```python
from build123d import *

# Parameters (mm, degrees)
SKETCH1_W           = 212.725
SKETCH1_H           = 185.42
BOSS_EXTRUDE1_DEPTH = 3.175
SKETCH5_W           = 3.175
SKETCH5_H           = 76.2
BOSS_EXTRUDE2_DEPTH = 3.175
SKETCH6_W           = 76.2
SKETCH6_H           = 3.175
BOSS_EXTRUDE3_DEPTH = 3.175


with BuildPart() as part:
    # Sketch1 → Boss-Extrude1 (new body)
    with BuildSketch(Plane.XY):
        Rectangle(SKETCH1_W, SKETCH1_H)
    extrude(amount=BOSS_EXTRUDE1_DEPTH)

    # Sketch5 → Boss-Extrude2 (add)
    with BuildSketch(Plane(origin=(0, 0, 0), x_dir=(-1, 0, 0), z_dir=(0, 0, -1))):
        with Locations((-107.95, 0)):
            Rectangle(SKETCH5_W, SKETCH5_H)
        with Locations((107.95, 0)):
            Rectangle(SKETCH5_W, SKETCH5_H)
    extrude(amount=-BOSS_EXTRUDE2_DEPTH)

    # Sketch6 → Boss-Extrude3 (add)
    with BuildSketch(Plane(origin=(0, 0, 0), x_dir=(-1, 0, 0), z_dir=(0, 0, -1))):
        with Locations((0, -94.2975)):
            Rectangle(SKETCH6_W, SKETCH6_H)
    extrude(amount=-BOSS_EXTRUDE3_DEPTH)


solid = part.part
```
For this review, take the finished solid that the model builds, in its own axes (mm). Coordinates: 2 decimals unless noted, no trailing zeros. Write each loop counter-clockwise with the first axis right and the second up, starting at its lowest first coordinate (ties: lowest second). Pieces come first, ordered by that corner, then holes. Notation, with made-up numbers: (13.25, 66) - (28.25, 66) arc R18 cw to (28.25, 88) - close; hole circle Ø7 at (-25, 26.5). An arc over 180 degrees is marked (long way). Answer in a Markdown table with one row per item. Add a question column.
Q1. Draft analysis for pull direction Z (two halves, no side actions). For faces 1 (the flat face through (-2, 0, 0)), 2 (the flat face through (-2, 0, 3.175)), state which applies: +Z half, -Z half, draft (parallel to the pull), parting line (faces both ways), or undercut.
Q2. We need section C-C, the plane x = 87.5. State the section outline as (y, z) points (3 decimals).
Q3. For probe 1 along Y at (x, z) = (-42.5, 2.6); probe 2 along X at (y, z) = (43.5, 1.45), list the stretches that pass through material, from the lowest coordinate up.
Q4. We need section A-A, the plane z = 1.9. State the section outline as (x, y) points (1 decimal), and give its area (3 significant figures).
Q5. We need section B-B, the plane y = 80. State the section outline as (x, z) points (1 decimal), and give its area (3 significant figures).
Q6. For P1, Ø1.6, axis at x = 108.5, z = 1.5, coming from the +Y side; P2, Ø1, axis at y = -78.5, z = 1, coming from the -X side; P3, Ø1, axis at x = -84, z = 2.5, coming from the -Y side, all flat-tipped, find the tip position at first contact; note any pin that passes through.
Answer list:
| question | item | result |
|---|---|---|
| 1 | face 1 | -Z half |
| 1 | face 2 | +Z half |
| 2 | outline | (-92.71, 0) - (92.71, 0) - (92.71, 3.175) - (-92.71, 3.175) - close |
| 3 | probe 1 | y = -92.71 to 92.71 |
| 3 | probe 2 | x = -106.36 to 106.36 |
| 4 | outline | (-109.5, -38.1) - (-106.4, -38.1) - (-106.4, -92.7) - (-38.1, -92.7) - (-38.1, -95.9) - (38.1, -95.9) - (38.1, -92.7) - (106.4, -92.7) - (106.4, -38.1) - (109.5, -38.1) - (109.5, 38.1) - (106.4, 38.1) - (106.4, 92.7) - (-106.4, 92.7) - (-106.4, 38.1) - (-109.5, 38.1) - close |
| 4 | area | 40,200 mm2 |
| 5 | outline | (-106.4, 0) - (106.4, 0) - (106.4, 3.2) - (-106.4, 3.2) - close |
| 5 | area | 675 mm2 |
| 6 | P1 | stops at y = 38.1 |
| 6 | P2 | stops at x = -106.36 |
| 6 | P3 | stops at y = -92.71 |
